For this review, take the finished solid that the model builds, in its own axes (mm). A direction names the side the tool comes from. Coordinates: 2 decimals unless noted, no trailing zeros. Write each loop counter-clockwise with the first axis right and the second up, starting at its lowest first coordinate (ties: lowest second). Pieces come first, ordered by that corner, then holes.
1) For faces 5 (the face through (-58, -36.6, -10)), 6 (the face through (-64.15, -48, -22)), 7 (the face through (-58, -33, -23)), 8 (the face through (-50.96, -35, -27.84)), list the 3-axis set-ups (+Z, -Z, +X, -X, +Y, -Y) from which the entire face can be reached by the end or side of a thin tool; tool diameter is ignored.
2) Mouldability with a two-part tool opening along X and no side actions: class faces 1 (the face through (-50.9, -47, -15.75)), 2 (the face through (-64.15, -48, -16)), 3 (the face through (-57.99, -47.96, -28.65)), 4 (the face through (-53.15, -48.4, -29.3)) as pulls with the +X half, pulls with the -X half, needs draft (parallel to the pull), parting line crosses it, or undercut.
3) To check wall thickness, follow line 1 along X through (y, z) = (-41.5, -16.5); line 2 along X through (y, z) = (-44, -13.75); line 3 along Y through (x, z) = (-55.5, -26). State the ranges of each line that lie inside material, in increasing order.
4) We need section B-B on z = -21.75. Write out the cut boundary in (x, y), then the cut area to 3 significant figures.
5) Insertion check: P1, Ø0.5, axis at x = -50.5, y = -52.5, coming from the -Z side; P2, Ø6, axis at y = -45.5, z = -12.5, coming from the -X side; P3, Ø0.9, axis at x = -51, y = -48.5, coming from the +Z side; P4, Ø12, axis at y = -49.5, z = -12, coming from the -X side. Each pin has a flat end and moves straight along its axis. Give the tip position at first contact, or say it passes through.
6) We need section D-D on z = -14.5. Write out the cut boundary in (x, y), then the cut area to 3 significant figures.
from build123d import *

# Parameters (mm, degrees)
SKETCH061_W        = 11.8
SKETCH061_H        = 25.8
SKETCH061_W_2      = 9.8
SKETCH061_H_2      = 23.8
PAD031_DEPTH       = 15
SKETCH062_W        = 15
SKETCH062_H        = 30.5
SKETCH062_W_2      = 9.8
SKETCH062_H_2      = 23.8
PAD032_DEPTH       = 1
SKETCH063_W        = 15
SKETCH063_H        = 30.5
SKETCH063_W_2      = 13
SKETCH063_H_2      = 28.5
PAD033_DEPTH       = 15
POCKET007016_DEPTH = 30.501
SKETCH065_W        = 15.029142
SKETCH065_H        = 29.5
PAD034_DEPTH       = 1
SKETCH066_W        = 26.5
SKETCH066_H        = 5
POCKET007017_DEPTH = 3


with BuildPart() as part:
    # Sketch061 → Pad031 (new body)
    with BuildSketch(Plane.XY):
        with Locations((-57.65, -16.5)):
            Rectangle(SKETCH061_W, SKETCH061_H)
        with Locations((-57.65, -16.5)):
            Rectangle(SKETCH061_W_2, SKETCH061_H_2, mode=Mode.SUBTRACT)
    extrude(amount=PAD031_DEPTH)

    # Sketch062 → Pad032 (join)
    with BuildSketch(Plane.XY):
        with Locations((-57.65, -16.25)):
            Rectangle(SKETCH062_W, SKETCH062_H)
        with Locations((-57.65, -16.5)):
            Rectangle(SKETCH062_W_2, SKETCH062_H_2, mode=Mode.SUBTRACT)
    extrude(amount=-PAD032_DEPTH)

    # Sketch063 (on DatumPlane) → Pad033 (join)
    with BuildSketch(Plane(origin=(0, 0, 1), x_dir=(-1, 0, 0), z_dir=(0, 0, -1))):
        with Locations((57.65, -16.25)):
            Rectangle(SKETCH063_W, SKETCH063_H)
        with Locations((57.65, -16.25)):
            Rectangle(SKETCH063_W_2, SKETCH063_H_2, mode=Mode.SUBTRACT)
    extrude(amount=PAD033_DEPTH)

    # Sketch064 (on DatumPlane) → Pocket007016 (cut, through all)
    with BuildSketch(Plane(origin=(-65.15, -31.5, 1), x_dir=(1, 0, 0), z_dir=(0, -1, 0))):
        Polygon((15, -15), (0, -10.980762), (0, -15), align=None)
    extrude(amount=-POCKET007016_DEPTH, mode=Mode.SUBTRACT)

    # Sketch065 (on Face37 of Pocket007016) → Pad034 (join)
    with BuildSketch(Plane(origin=(-6.859413, 0, -25.599678), x_dir=(0.965926, 0, -0.258819), z_dir=(-0.258819, 0, -0.965926))):
        with Locations((-52.832285, 15.75)):
            Rectangle(SKETCH065_W, SKETCH065_H)
    extrude(amount=-PAD034_DEPTH)

    # Sketch066 (on Face36 of Pad034) → Pocket007017 (cut)
    with BuildSketch(Plane.YZ.offset(-50.15)):
        with Locations((-16.25, -10.5)):
            Rectangle(SKETCH066_W, SKETCH066_H)
    extrude(amount=-POCKET007017_DEPTH, mode=Mode.SUBTRACT)


with BuildPart() as part_1:
    # Body004 placement: moved
    add(part.part.moved(Location((0, -32, -16.75))))


solid = part_1.part
Result:
1. face 5: +Z
1. face 6: none
1. face 7: +Z, -Z, +X, -X, +Y
1. face 8: +X
2. face 1: needs draft
2. face 2: undercut
2. face 3: pulls with the -X half
2. face 4: pulls with the +X half
3. line 1: x = -65.15 to -64.15, -63.55 to -62.55, -52.75 to -51.75, -51.15 to -50.15
3. line 2: x = -63.55 to -62.55, -52.75 to -51.75
3. line 3: y = -63.5 to -62.5, -34 to -33
4. outline: (-65.15, -63.5) - (-50.15, -63.5) - (-50.15, -33) - (-65.15, -33) - close; hole (-64.15, -62.5) - (-51.15, -62.5) - (-51.15, -34) - (-64.15, -34) - close
4. area: 87.0 mm2
5. P1: stops at z = -30.72
5. P2: stops at x = -63.55
5. P3: stops at z = -15.75
5. P4: stops at x = -65.15
6. outline: (-63.55, -61.4) - (-51.75, -61.4) - (-51.75, -35.6) - (-63.55, -35.6) - close; hole (-62.55, -60.4) - (-52.75, -60.4) - (-52.75, -36.6) - (-62.55, -36.6) - close
6. area: 71.2 mm2
